Part print with two shaded views. Sizes in mm from the minimum x, y, z corner. Coordinates: 2 decimals unless noted, no trailing zeros.
Item 1: Flat gauge pin, fed straight in: pin 1 (4.5 mm diameter, centred on x = 315, y = 5, fed in from -Z). Where does the tip first touch, or does it go through?
Item 2: Drill centre lines: line 1 along Y through (x, z) = (5, 1.8); line 2 along Y through (x, z) = (237.5, 3.3). Where is each one in solid material? Low to high.
Item 3: Cut at A-A (z = 1.75). Count the separate pieces of the cut face and the enclosed holes in it, and give its area (3 significant figures).
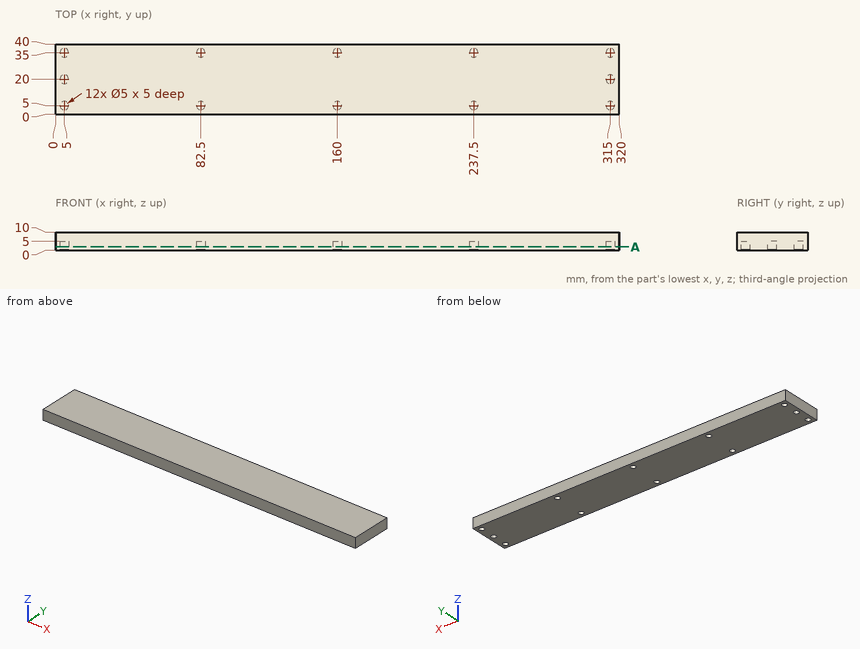
Filled sheet:
1. pin 1: stops at z = 5
2. line 1: y = 0 to 2.5, 7.5 to 17.5, 22.5 to 32.5, 37.5 to 40
2. line 2: y = 0 to 2.5, 7.5 to 32.5, 37.5 to 40
3. separate pieces: 1
3. enclosed holes: 12
3. area: 12,600 mm2
